```python
from build123d import *

# Parameters (mm, degrees)
SKETCH_1_W                   = 100
SKETCH_1_H                   = 100
EXTRUDE_1_DEPTH              = 15
HOLE_WIZARD_M6_1_D           = 6.4
HOLE_WIZARD_M6_1_CBORE_D     = 11
HOLE_WIZARD_M6_1_CBORE_DEPTH = 6.4
SKETCH_4_R                   = 30
CUT_EXTRUDE_1_DEPTH          = 5
HOLE_WIZARD_M6_2_D           = 6.4
HOLE_WIZARD_M6_2_CBORE_D     = 11
HOLE_WIZARD_M6_2_CBORE_DEPTH = 6.4
SKETCH_8_R                   = 25
CUT_EXTRUDE_2_DEPTH          = 11


with BuildPart() as part:
    # 草图1 → 凸台-拉伸1 (new body)
    with BuildSketch(Plane.XY):
        Rectangle(SKETCH_1_W, SKETCH_1_H)
    extrude(amount=EXTRUDE_1_DEPTH)

    # M6 六角凹头螺钉的柱形沉头孔1 (through all)
    with Locations(Plane(origin=(-40, 40, 0), x_dir=(-1, 0, 0), z_dir=(0, 0, -1))):
        with Locations((0, 0), (-80, 0), (-80, -80), (0, -80)):
            CounterBoreHole(HOLE_WIZARD_M6_1_D / 2, HOLE_WIZARD_M6_1_CBORE_D / 2, HOLE_WIZARD_M6_1_CBORE_DEPTH)

    # 草图4 → 切除-拉伸1 (cut)
    with BuildSketch(Plane.XY):
        Circle(SKETCH_4_R)
    extrude(amount=CUT_EXTRUDE_1_DEPTH, mode=Mode.SUBTRACT)

    # M6 六角凹头螺钉的柱形沉头孔2 (through all)
    with Locations(Plane(origin=(-24.748737342, 24.748737342, 15), x_dir=(1, 0, 0), z_dir=(0, 0, 1))):
        with Locations((0, 0), (0, -49.497474684), (49.497474684, -49.497474684), (49.497474684, 0)):
            CounterBoreHole(HOLE_WIZARD_M6_2_D / 2, HOLE_WIZARD_M6_2_CBORE_D / 2, HOLE_WIZARD_M6_2_CBORE_DEPTH)

    # 草图8 → 切除-拉伸2 (cut, through all)
    with BuildSketch(Plane(origin=(0, 0, 5), x_dir=(-1, 0, 0), z_dir=(0, 0, -1))):
        Circle(SKETCH_8_R)
    extrude(amount=-CUT_EXTRUDE_2_DEPTH, mode=Mode.SUBTRACT)


solid = part.part
```
CAD build for the part. Positions are in the model's coordinates, mm. A direction names the side the tool comes from. Coordinates: 2 decimals unless noted, no trailing zeros. Loops run counter-clockwise (first coordinate to the right, second up) from the corner with the lowest first, then second, coordinate; pieces in that order, holes last. Notation, with made-up numbers: (5, -27.5) - (46, -27.5) arc R24 cw to (46, 7.5) - close; hole circle Ø8 at (34.25, -3.75). An arc over 180 degrees is marked (long way). Return JSON: item names as keys, results as strings.
1. Drop a flat-ended pin along its axis: pin 1 (5.5 mm diameter, centred on x = -38.5, y = 39.5, fed in from -Z). Give the stop position or say it passes through.
Result:
{"pin 1": "stops at z = 6.4"}
2. Mould opens along X. For faces 4 (the cylindrical face through (23.56, 19.38, 11.84)), 5 (the cylindrical face through (39.583, 43.173, 10.76)), 6 (the flat face through (-12, 23, 15)), 7 (the flat face through (-50, -1, 7)) say: released by +X, released by -X, zero draft, split by the parting line, or undercut.
Result:
{"face 4": "undercut", "face 5": "undercut", "face 6": "zero draft", "face 7": "released by -X"}
3. 3-axis set-ups, long thin cutter, end or side, ignore diameter. For faces 1 (the cylindrical face through (-25.94, 19.38, 11.84)), 2 (the flat face through (-1, 50, 7)), 3 (the flat face through (-7, 25, 5)): which of +Z, -Z, +X, -X, +Y, -Y reach the whole face in a straight line?
Result:
{"face 1": "+Z", "face 2": "+Z, -Z, +X, -X, +Y", "face 3": "-Z"}
4. Band-saw the part on A-A (y = -40). Give the cut face in (x, z), and give its area (3 significant figures).
Result:
{"outline": "(-50, 0) - (-45.5, 0) - (-45.5, 6.4) - (-43.2, 6.4) - (-43.2, 15) - (-50, 15) - close; (-36.8, 6.4) - (-34.5, 6.4) - (-34.5, 0) - (34.5, 0) - (34.5, 6.4) - (36.8, 6.4) - (36.8, 15) - (-36.8, 15) - close; (43.2, 6.4) - (45.5, 6.4) - (45.5, 0) - (50, 0) - (50, 15) - (43.2, 15) - close", "area": "1,250 mm2"}
5. Band-saw the part on C-C (x = 0). Give the cut face in (y, z).
Result:
{"outline": "(-50, 0) - (-30, 0) - (-30, 5) - (-25, 5) - (-25, 15) - (-50, 15) - close; (25, 5) - (30, 5) - (30, 0) - (50, 0) - (50, 15) - (25, 15) - close"}
6. Probe L1, parallel to Y at x = -40, z = 12.25; L2, parallel to Y at x = 40, z = 5; L3, parallel to X at y = -8, z = 11. List the from-to ranges inside material, lowest first. Write a range as from..to.
Result:
{"L1": "y = -50..-43.2, -36.8..36.8, 43.2..50", "L2": "y = -50..-45.5, -34.5..34.5, 45.5..50", "L3": "x = -50..-23.69, 23.69..50"}
